Input: part model. Units: mm. Frame: model coordinates. Coordinates: 2 decimals unless noted, no trailing zeros. Write each loop counter-clockwise with the first axis right and the second up, starting at its lowest first coordinate (ties: lowest second). Pieces come first, ordered by that corner, then holes. Notation, with made-up numbers: (52, 4.25) - (74, 4.25) arc R6 cw to (74, 13.25) - close; hole circle Ø4 at (32, -2). An arc over 180 degrees is marked (long way). Put each result on its own line as item: value. Start each with the question number.
1. Line query: line 1 (Z direction, x = 22.5, y = 0.15); line 2 (X direction, y = 1.85, z = 49.5); line 3 (X direction, y = 0.3, z = -50). Output: solid intervals per line, ascending.
2. Cut plane B-B, the plane z = 50. Return loops of the section in (x, y).
3. Cut plane A-A, the plane y = 1.2. Return loops of the section in (x, z), and give its area (3 significant figures).
4. Cut plane C-C, the plane x = -31.5. Return loops of the section in (y, z), and give its area (3 significant figures).
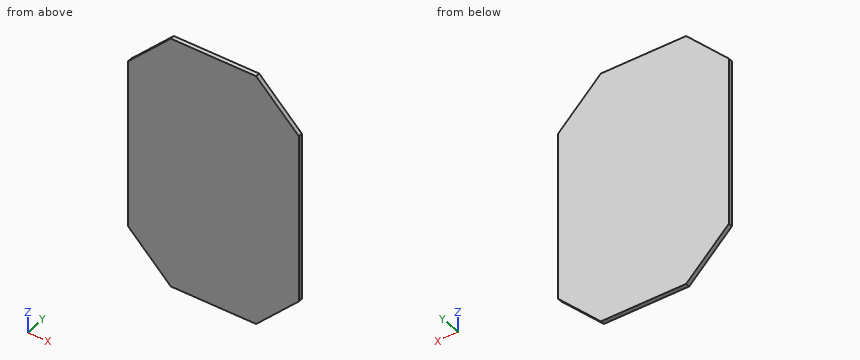
from build123d import *

# Parameters (mm, degrees)
SKETCH1_W           = 80
SKETCH1_H           = 80
BOSS_EXTRUDE1_DEPTH = 2


with BuildPart() as part:
    # Sketch1 → Boss-Extrude1 (new body)
    with BuildSketch(Plane(origin=(0, 0, 0), x_dir=(1, 0, 0), z_dir=(0, 1, 0))):
        Rectangle(SKETCH1_W, SKETCH1_H)
        Polygon((20, 60), (40, 40), (-40, 40), (-20, 60), align=None)
        Polygon((-40, -40), (40, -40), (20, -60), (-20, -60), align=None)
    extrude(amount=BOSS_EXTRUDE1_DEPTH)


solid = part.part
Report:
1. line 1: z = -57.5 to 57.5
1. line 2: x = -30.5 to 30.5
1. line 3: x = -30 to 30
2. outline: (-30, 0) - (30, 0) - (30, 2) - (-30, 2) - close
3. outline: (-40, -40) - (-20, -60) - (20, -60) - (40, -40) - (40, 40) - (20, 60) - (-20, 60) - (-40, 40) - close
3. area: 8,800 mm^2
4. outline: (0, -48.5) - (2, -48.5) - (2, 48.5) - (0, 48.5) - close
4. area: 194 mm^2
